Source: three-view drawing plus pictorial views. Frame: mm from the lowest corner of the part. A direction names the side the tool comes from. Give positions to 0.01 mm unless a question says otherwise; leave off trailing zeros. Write each loop counter-clockwise with the first axis right and the second up, starting at its lowest first coordinate (ties: lowest second). Pieces come first, ordered by that corner, then holes.
Q1. Line query: L1, parallel to X at y = 3.05, z = 14; L2, parallel to Z at x = 9.5, y = 2.35. Output: solid intervals per line, ascending.
Q2. Reachability of the marked faces 1 and 2 from +Z, -Z, +X, -X, +Y, -Y: full face, straight path, thin tool, end or side. Return the list, or none.
Q3. Pin query (flat end, axial travel): pin 1 (3 mm diameter, centred on x = 1, y = 1.5, fed in from -Z); pin 2 (2.5 mm diameter, centred on y = 1.5, z = 3, fed in from -X); pin 3 (1.5 mm diameter, centred on y = 2, z = 1.5, fed in from +X). Return the tip coordinate at first contact, or that it passes through.
Q4. Cut plane B-B on z = 18. Return the cut outline in (x, y), plus the area to 3 significant figures.
Q5. Cut plane A-A on y = 3.8. Count the separate pieces of the cut face and the enclosed holes in it, plus the area to 3 significant figures.
Q6. Cut plane C-C on x = 1.25. Return the cut outline in (y, z), plus the area to 3 significant figures.
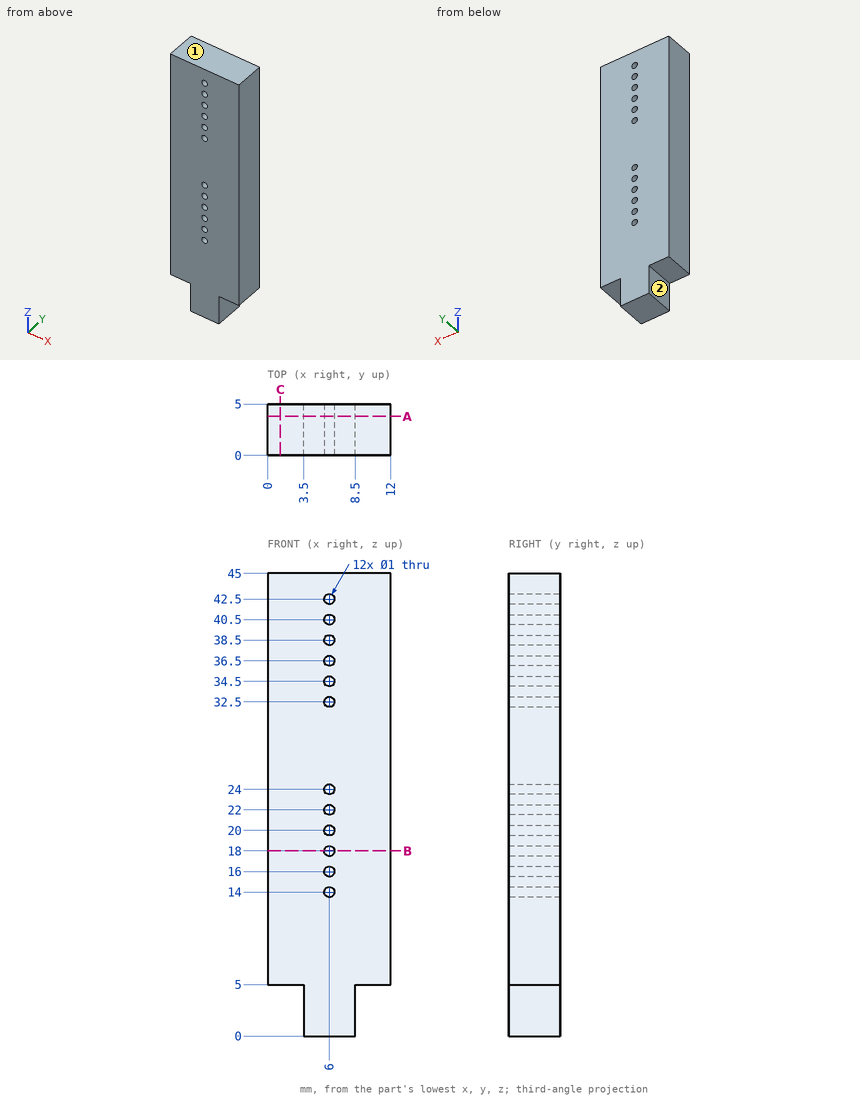
Data:
1. L1: x = 0 to 5.5, 6.5 to 12
1. L2: z = 5 to 45
2. face 1: +Z, +X, -X, +Y, -Y
2. face 2: -Z, -X, +Y, -Y
3. pin 1: stops at z = 5
3. pin 2: stops at x = 3.5
3. pin 3: stops at x = 8.5
4. outline: (0, 0) - (5.5, 0) - (5.5, 5) - (0, 5) - close; (6.5, 0) - (12, 0) - (12, 5) - (6.5, 5) - close
4. area: 55.0 mm2
5. separate pieces: 1
5. enclosed holes: 12
5. area: 496 mm2
6. outline: (0, 5) - (5, 5) - (5, 45) - (0, 45) - close
6. area: 200 mm2
